```python
from build123d import *

# Parameters (mm, degrees)
SKETCH1_R               = 6
SKETCH1_R_2             = 5
EXTRUDE_THIN1_DEPTH     = 100
SKETCH2_R               = 1.5
CUT_EXTRUDE2_DEPTH      = 7
CUT_EXTRUDE2_DEPTH_BACK = 7
SKETCH3_R               = 1.5
CUT_EXTRUDE3_DEPTH      = 7.000000127
CUT_EXTRUDE3_DEPTH_BACK = 7.000000127


with BuildPart() as part:
    # Sketch1 → Extrude-Thin1 (new body)
    with BuildSketch(Plane(origin=(0, 0, 0), x_dir=(1, 0, 0), z_dir=(0, 1, 0))):
        Circle(SKETCH1_R)
        Circle(SKETCH1_R_2, mode=Mode.SUBTRACT)
    extrude(amount=EXTRUDE_THIN1_DEPTH)

    # Sketch2 → Cut-Extrude2 (cut, two sides)
    with BuildSketch(Plane.XY) as cut_extrude2_sk:
        with Locations((0, 8)):
            Circle(SKETCH2_R)
    extrude(amount=CUT_EXTRUDE2_DEPTH, mode=Mode.SUBTRACT)
    extrude(cut_extrude2_sk.sketch, amount=-CUT_EXTRUDE2_DEPTH_BACK, mode=Mode.SUBTRACT)

    # Sketch3 → Cut-Extrude3 (cut, two sides)
    with BuildSketch(Plane.XY) as cut_extrude3_sk:
        with Locations((0, 92)):
            Circle(SKETCH3_R)
    extrude(amount=CUT_EXTRUDE3_DEPTH, mode=Mode.SUBTRACT)
    extrude(cut_extrude3_sk.sketch, amount=-CUT_EXTRUDE3_DEPTH_BACK, mode=Mode.SUBTRACT)


solid = part.part
```
Here's how the part is built. I have some questions about the finished solid (model axes, mm). Coordinates: 2 decimals unless noted, no trailing zeros. Write each loop counter-clockwise with the first axis right and the second up, starting at its lowest first coordinate (ties: lowest second). Pieces come first, ordered by that corner, then holes. Notation, with made-up numbers: (64, 20) - (103, 20) arc R10 cw to (103, 32) - close; hole circle Ø2 at (-24, -11). An arc over 180 degrees is marked (long way). One line per item, written item: value.
1) Suppose I cut it at D-D on y = 78. Write out the boundary of the cut face in (x, z), and give its area (3 significant figures).
Model answer:
outline: circle Ø12 at (0, 0); hole circle Ø10 at (0, 0)
area: 34.6 mm²
2) Suppose I cut it at B-B on x = 0. Write out the boundary of the cut face in (y, z), and give its area (3 significant figures).
Model answer:
outline: (0, -6) - (6.5, -6) - (6.5, -5) - (0, -5) - close; (0, 5) - (6.5, 5) - (6.5, 6) - (0, 6) - close; (9.5, -6) - (90.5, -6) - (90.5, -5) - (9.5, -5) - close; (9.5, 5) - (90.5, 5) - (90.5, 6) - (9.5, 6) - close; (93.5, -6) - (100, -6) - (100, -5) - (93.5, -5) - close; (93.5, 5) - (100, 5) - (100, 6) - (93.5, 6) - close
area: 188 mm²
3) I need wall thicknesses on line 1 along Y through (x, z) = (0, 5.3); line 2 along Z through (x, y) = (0.25, 43.5); line 3 along Y through (x, z) = (-0.75, 5.5). Which ranges of each line are inside material? Lowest first, please.
Model answer:
line 1: y = 0 to 6.5, 9.5 to 90.5, 93.5 to 100
line 2: z = -5.99 to -4.99, 4.99 to 5.99
line 3: y = 0 to 6.7, 9.3 to 90.7, 93.3 to 100
4) Suppose I cut it at C-C on y = 92. Write out the boundary of the cut face in (x, z).
Model answer:
outline: (-1.5, -5.81) - (-1.5, -4.77) arc R5 cw to (-1.5, 4.77) - (-1.5, 5.81) arc R6 ccw to start; (1.5, -5.81) arc R6 ccw to (1.5, 5.81) - (1.5, 4.77) arc R5 cw to (1.5, -4.77) - close
5) I'm going to push flat-ended pins straight in: P1, Ø2.5, axis at x = 0, y = 8, coming from the +Z side; P2, Ø5, axis at x = -4.5, y = 85, coming from the -Z side; P3, Ø3, axis at y = 33, z = 4.5, coming from the +X side; P4, Ø2, axis at y = 88.5, z = 2, coming from the -X side. Where does each tip first touch, or does it pass through?
Model answer:
P1: passes through
P2: stops at z = -5.66
P3: stops at x = 5.2
P4: stops at x = -5.92
6) We'd pull the mould along Y, two halves only. Please class faces 1 (the flat face through (-4, 0, -4)), 2 (the flat face through (-4, 100, -4)), 3 (the cylindrical face through (1.43, 92.45, -5.38)), 4 (the cylindrical face through (-1.08, 49.3, 4.88)): pulls with the +Y half, pulls with the -Y half, needs draft (parallel to the pull), parting line crosses it, or undercut.
Model answer:
face 1: pulls with the -Y half
face 2: pulls with the +Y half
face 3: undercut
face 4: needs draft
7) Suppose I cut it at A-A on z = 0. Write out the boundary of the cut face in (x, y).
Model answer:
outline: (-6, 0) - (-5, 0) - (-5, 100) - (-6, 100) - close; (5, 0) - (6, 0) - (6, 100) - (5, 100) - close
